CAD build for the part. Positions are in the model's coordinates, mm. A direction names the side the tool comes from. Coordinates: 2 decimals unless noted, no trailing zeros. Order: outer loops, then holes, each group sorted by start corner. A loop starts at its lowest first (then second) coordinate and runs counter-clockwise, first axis right, second up.
from build123d import *

# Parameters (mm, degrees)
SKETCH1_R            = 5
BOSS_EXTRUDE9_DEPTH  = 40
SKETCH6_W            = 49.606003438
SKETCH6_H            = 60
SKETCH6_H_2          = 6
CUT_EXTRUDE5_DEPTH   = 40
BOSS_EXTRUDE11_DEPTH = 40
SKETCH7_W            = 22
SKETCH7_H            = 29.796679389
CUT_EXTRUDE6_DEPTH   = 80
BOSS_EXTRUDE12_DEPTH = 40


with BuildPart() as part:
    # Sketch1 → Boss-Extrude9 (new, symmetric)
    with BuildSketch(Plane.XY):
        with BuildLine():
            ThreePointArc((16, 13), (34.941864918, 22.051658235), (49.606003438, 37.074634133))
            Line((49.606003438, 37.074634133), (44, 41))
            Line((44, 41), (5, 41))
            Line((5, 41), (0, 36))
            Line((0, 36), (0, 13))
            Line((0, 13), (16, 13))
        make_face()
        with Locations((12, 31)):
            Circle(SKETCH1_R, mode=Mode.SUBTRACT)
    extrude(amount=BOSS_EXTRUDE9_DEPTH, both=True)

    # Sketch6 → Cut-Extrude5 (cut)
    with BuildSketch(Plane(origin=(0, 41, 0), x_dir=(1, 0, 0), z_dir=(0, 1, 0))):
        with Locations((24.803001719, 0)):
            Rectangle(SKETCH6_W, SKETCH6_H)
        with Locations((24.803001719, -37)):
            Rectangle(SKETCH6_W, SKETCH6_H_2)
    extrude(amount=-CUT_EXTRUDE5_DEPTH, mode=Mode.SUBTRACT)


with BuildPart() as cut_extrude5_piece_1:
    # of the separate pieces the step leaves, piece 1, a body of its own (cut_extrude5_pieces)
    add(part.part.solids().sort_by_distance((16, 13, -30))[0])



with BuildPart() as cut_extrude5_piece_2:
    # of the separate pieces the step leaves, piece 2, a body of its own (cut_extrude5_pieces)
    add(part.part.solids().sort_by_distance((16, 13, 34))[0])


with BuildPart() as body_3:
    # Sketch1<13> → Boss-Extrude11 (new, symmetric)
    with BuildSketch(Plane.XY):
        Polygon((65, 26.295641698), (60, 29.796679389), (60, 5), (0, 5), (0, 0), (65, 0), align=None)
    extrude(amount=BOSS_EXTRUDE11_DEPTH, both=True)

    # Sketch7 → Cut-Extrude6 (cut)
    with BuildSketch(Plane(origin=(65, 0, 0), x_dir=(0, 0, -1), z_dir=(1, 0, 0))):
        with Locations((2.518815971, 14.898339695)):
            Rectangle(SKETCH7_W, SKETCH7_H)
    extrude(amount=-CUT_EXTRUDE6_DEPTH, mode=Mode.SUBTRACT)


with BuildPart() as cut_extrude6_piece_1:
    # of the separate pieces the step leaves, piece 1, a body of its own (cut_extrude6_pieces)
    add(body_3.part.solids().sort_by_distance((65, 26.295641698, 40))[0])


with BuildPart() as cut_extrude6_piece_2:
    # of the separate pieces the step leaves, piece 2, a body of its own (cut_extrude6_pieces)
    add(body_3.part.solids().sort_by_distance((65, 26.295641698, -13.518815971))[0])


with BuildPart() as cut_extrude5_piece_1_1:
    add(cut_extrude5_piece_1.part)

    add(cut_extrude5_piece_2.part)  # Boss-Extrude12 merges Cut-Extrude5 piece 2

    add(cut_extrude6_piece_1.part)  # Boss-Extrude12 merges Cut-Extrude6 piece 1

    add(cut_extrude6_piece_2.part)  # Boss-Extrude12 merges Cut-Extrude6 piece 2
    # Sketch1<14> → Boss-Extrude12 (add, symmetric)
    with BuildSketch(Plane.XY):
        with BuildLine():
            Line((60, 5), (60, 29.796679389))
            Line((60, 29.796679389), (49.606003438, 37.074634133))
            ThreePointArc((49.606003438, 37.074634133), (34.941864918, 22.051658235), (16, 13))
            Line((16, 13), (0, 13))
            Line((0, 13), (0, 5))
            Line((0, 5), (60, 5))
        make_face()
    extrude(amount=BOSS_EXTRUDE12_DEPTH, both=True)


solid = cut_extrude5_piece_1_1.part
1) Slice it at B-B (z = -27.5). List the corners of the cut face in (x, y), plus the area to 3 significant figures.
2) Two-plate mould, pull along Z, no slides. Class faces 6 (the flat face through (32, 21, -40)), 7 (the flat face through (19, 27, 34)), 8 (the flat face through (37, 4, 8.481)), 9 (the flat face through (32, 0, -27)): released by +Z, released by -Z, zero draft, split by the parting line, or undercut.
3) Slice it at A-A (x = 12). List the corners of the cut face in (y, z).
4) Drill centre lines: probe 1 along Y at (x, z) = (12, -34.5); probe 2 along Z at (x, y) = (9.5, 14.5); probe 3 along Z at (x, y) = (59, 3.5). Where is each one in solid material? Low to high.
5) Slice it at C-C (y = 31). List the corners of the cut face in (x, z).
6) Which spindle directions (+Z, -Z, +X, -X, +Y, -Y) get a long thin tool onto all of the face, cutting with end or side? Do faces 1 (the flat face through (60, 17, -2)), 2 (the flat face through (8, 13, 0)), 3 (the flat face through (8, 13, 37)), 4 (the flat face through (30, 5, -2)), 5 (the flat face through (37, 4, -13.519)). Say none if no direction does.
7) Pin check, flat tips, straight feed: P1, Ø10, axis at x = 39.5, z = -2, coming from the -Y side; P2, Ø4, axis at x = 13.5, z = 23, coming from the +Y side; P3, Ø3, axis at y = 32, z = -3.5, coming from the -X side. Stop position of each tip, or through.
8) Slice it at D-D (y = 21.5). List the corners of the cut face in (x, z).
Worked out:
1. outline: (0, 0) - (65, 0) - (65, 26.3) - (49.61, 37.07) arc R60 cw to (16, 13) - (0, 13) - close
1. area: 1,440 mm2
2. face 6: released by -Z
2. face 7: released by +Z
2. face 8: undercut
2. face 9: zero draft
3. outline: (0, -40) - (26, -40) - (26, -30) - (13, -30) - (13, 30) - (26, 30) - (26, 34) - (13, 34) - (13, 40) - (0, 40) - (0, 8.48) - (5, 8.48) - (5, -13.52) - (0, -13.52) - close; (36, -40) - (41, -40) - (41, -30) - (36, -30) - close; (36, 30) - (41, 30) - (41, 34) - (36, 34) - close
4. probe 1: y = 0 to 26, 36 to 41
4. probe 2: z = -40 to -30, 30 to 34
4. probe 3: z = -40 to -13.52, 8.48 to 40
5. outline: (0, -40) - (7, -40) - (7, -30) - (0, -30) - close; (0, 30) - (7, 30) - (7, 34) - (0, 34) - close; (17, -40) - (58.28, -40) - (58.28, 40) - (44.88, 40) - (44.88, 34) - (17, 34) - (17, 30) - (44.88, 30) - (44.88, -30) - (17, -30) - close
6. face 1: +X, +Y, -Y
6. face 2: -X, +Y
6. face 3: +Z, -X, +Y
6. face 4: +X, -X, -Y
6. face 5: +X, -Y
7. P1: stops at y = 5
7. P2: stops at y = 13
7. P3: stops at x = 44.43
8. outline: (0, -40) - (65, -40) - (65, -13.52) - (60, -13.52) - (60, 8.48) - (65, 8.48) - (65, 40) - (34.16, 40) - (34.16, 34) - (0, 34) - (0, 30) - (34.16, 30) - (34.16, -30) - (0, -30) - close
